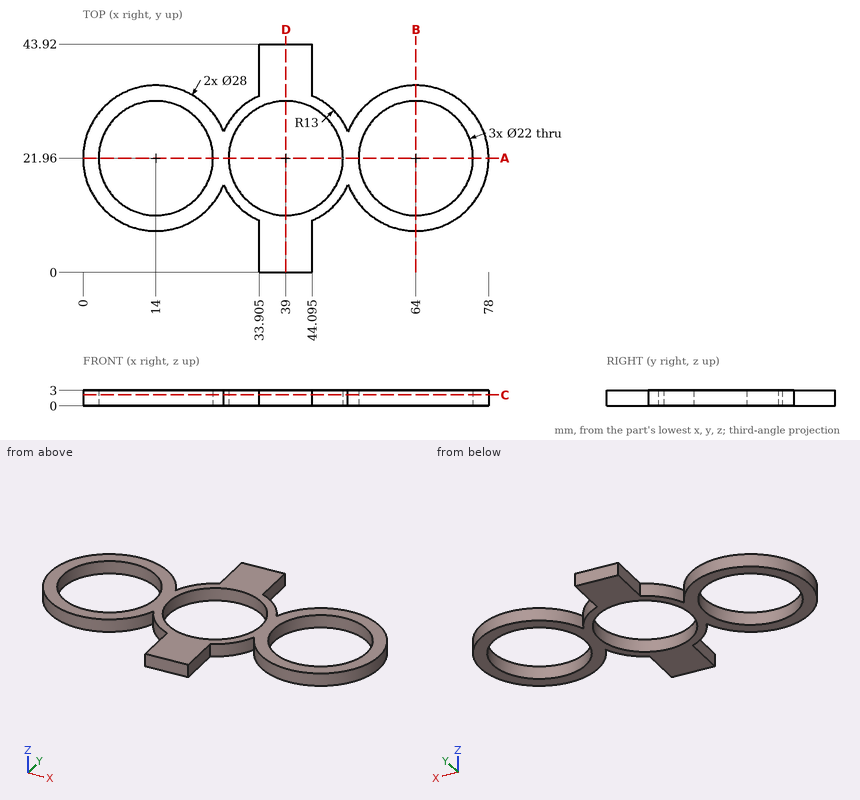
Geometry check sheet. Reference: drawing and pictorial views, mm from the part's lowest x, y, z. Coordinates: 2 decimals unless noted, no trailing zeros. Write each loop counter-clockwise with the first axis right and the second up, starting at its lowest first coordinate (ties: lowest second). Pieces come first, ordered by that corner, then holes. Notation, with made-up numbers: M 10.25,23.25 L 54.25,23.25 A26 ccw 54.25,40.25 Z; hole C 16.25,-4.5 d10. An arc over 180 degrees is marked long. Use one line per item in the form item = value.
Item 1: Sectioned sample at A-A, the plane y = 21.96. Record the cut outline in (x, z).
Answer below:
outline = M 0,0 L 3,0 L 3,3 L 0,3 Z; M 25,0 L 28,0 L 28,3 L 25,3 Z; M 50,0 L 53,0 L 53,3 L 50,3 Z; M 75,0 L 78,0 L 78,3 L 75,3 Z
Item 2: Sectioned sample at D-D, the plane x = 39. Record the cut outline in (y, z).
Answer below:
outline = M 0,0 L 10.96,0 L 10.96,3 L 0,3 Z; M 32.96,0 L 43.92,0 L 43.92,3 L 32.96,3 Z
Item 3: Gauge pin test, flat ends, axial feed: pin 1 Ø0.9 at (y, z) = (39, 1) entering from -X (3 decimals); pin 2 Ø1.5 at (y, z) = (4.5, 2) entering from +X (3 decimals); pin 3 Ø1 at (y, z) = (29.5, 2) entering from -X. Record the tip position at first contact, or that the pin passes through.
Answer below:
pin_1 = 33.905
pin_2 = 44.095
pin_3 = 1.9
Item 4: Sectioned sample at C-C, the plane z = 2.15. Record the cut outline in (x, y) (3 decimals), and give its area (3 significant figures).
Answer below:
outline = M 27.04,16.865 A13 ccw 33.905,10 L 33.905,0 L 44.095,0 L 44.095,10 A13 ccw 50.96,16.865 A14 ccw long 50.96,27.055 A13 ccw 44.095,33.92 L 44.095,43.92 L 33.905,43.92 L 33.905,33.92 A13 ccw 27.04,27.055 A14 ccw long Z; hole C 14,21.96 d22; hole C 39,21.96 d22; hole C 64,21.96 d22
area = 784 mm^2
Item 5: Material ranges on L1, parallel to Y at x = 39, z = 1.6; L2, parallel to Y at x = 14, z = 1.1; L3, parallel to X at y = 18.5, z = 1.7, recorded low to high. Write a range as from..to.
Answer below:
L1 = 0..10.96, 32.96..43.92
L2 = 7.96..10.96, 32.96..35.96
L3 = 0.43..3.56, 24.44..28.56, 49.44..53.56, 74.44..77.57
Item 6: Sectioned sample at B-B, the plane x = 64. Record the cut outline in (y, z).
Answer below:
outline = M 7.96,0 L 10.96,0 L 10.96,3 L 7.96,3 Z; M 32.96,0 L 35.96,0 L 35.96,3 L 32.96,3 Z
